The model under review builds one solid part; all positions refer to its coordinate system, in mm. A direction names the side the tool comes from. Coordinates: 2 decimals unless noted, no trailing zeros. Order: outer loops, then holes, each group sorted by start corner. A loop starts at its lowest first (then second) coordinate and runs counter-clockwise, first axis right, second up.
from build123d import *

# Parameters (mm, degrees)
EXTRUDE_1_DEPTH             = 15
HOLE_WIZARD_M121_D          = 10.2
HOLE_WIZARD_M121_DEPTH      = 15
HOLE_WIZARD_M61_D           = 5
HOLE_WIZARD_M61_DEPTH       = 15
HOLE_WIZARD_5_5_5_5_1_D     = 5.5
HOLE_WIZARD_5_5_5_5_1_DEPTH = 15
SKETCH_9_W                  = 6
SKETCH_9_H                  = 6
SKETCH_9_H_2                = 3
SKETCH_9_W_2                = 3
EXTRUDE_2_DEPTH             = 2
FILLET_1_R                  = 2


with BuildPart() as part:
    # Эскиз1 → Бобышка-Вытянуть1 (new body)
    with BuildSketch(Plane(origin=(0, 0, 0), x_dir=(1, 0, 0), z_dir=(0, 1, 0))):
        Polygon((0, 0), (0, 90), (30, 90), (90, 30), (90, 0), align=None)
    extrude(amount=EXTRUDE_1_DEPTH)

    # Отверстие обработанное метчиком M121
    with Locations(Plane(origin=(0, 15, 0), x_dir=(1, 0, 0), z_dir=(0, 1, 0))):
        with Locations((45, 45)):
            Hole(HOLE_WIZARD_M121_D / 2, depth=HOLE_WIZARD_M121_DEPTH)

    # Отверстие обработанное метчиком M61
    with Locations(Plane(origin=(0, 15, 0), x_dir=(1, 0, 0), z_dir=(0, 1, 0))):
        with Locations((37.928932188, 73.284271247), (73.284271247, 37.928932188), (52.071067812, 16.715728753), (16.715728753, 52.071067812)):
            Hole(HOLE_WIZARD_M61_D / 2, depth=HOLE_WIZARD_M61_DEPTH)

    # Диаметр отверстия Ø5.5 (5.5)1
    with Locations(Plane(origin=(0, 15, 0), x_dir=(1, 0, 0), z_dir=(0, 1, 0))):
        with Locations((15, 75), (15, 40), (15, 15), (40, 15), (75, 15)):
            Hole(HOLE_WIZARD_5_5_5_5_1_D / 2, depth=HOLE_WIZARD_5_5_5_5_1_DEPTH)

    # Эскиз9 → Бобышка-Вытянуть2 (add)
    with BuildSketch(Plane(origin=(0, 15, 0), x_dir=(1, 0, 0), z_dir=(0, 1, 0))):
        with Locations((15, 83)):
            Rectangle(SKETCH_9_W, SKETCH_9_H)
        with Locations((15, 60.071067812)):
            Rectangle(SKETCH_9_W, SKETCH_9_H)
        with Locations((15, 32)):
            Rectangle(SKETCH_9_W, SKETCH_9_H_2)
        with Locations((32, 15)):
            Rectangle(SKETCH_9_W_2, SKETCH_9_H)
        with Locations((60.071067812, 15)):
            Rectangle(SKETCH_9_W, SKETCH_9_H)
        with Locations((83, 15)):
            Rectangle(SKETCH_9_W, SKETCH_9_H)
    extrude(amount=EXTRUDE_2_DEPTH)

    # Скругление1
    fillet_1_edges = [part.edges().sort_by_distance(p)[0] for p in [
        (0, 7.5, 0),
        (0, 7.5, -90),
        (30, 7.5, -90),
        (90, 7.5, -30),
        (90, 7.5, 0),
    ]]
    fillet(fillet_1_edges, radius=FILLET_1_R)


solid = part.part
(1) Wall thickness on line 1 (X direction, y = 7.25, z = -15); line 2 (Z direction, x = 15, y = 3); line 3 (Y direction, x = 37.5, z = -39.5): over which ranges is each line inside the solid? List them lowest first.
(2) Insertion check: pin 1 Ø2 at (y, z) = (16.5, -14.5) entering from +X; pin 2 Ø8 at (x, z) = (16.72, -52.07) entering from +Y; pin 3 Ø0.6 at (x, y) = (15.5, 16) entering from +Z. Each pin has a flat end and moves straight along its axis. Give the tip position at first contact, or say it passes through.
(3) Consider section B-B (x = 41.5). Give the boundary of the cut face in (y, z).
(4) Consider section D-D (x = 59). Give the boundary of the cut face in (y, z).
(5) The part is to be moulded in two halves that separate along Z. For faces 1 (the face through (60, 7, -60)), 2 (the face through (15.358, 7.395, -17.727)), 3 (the face through (15.358, 7.395, -42.727)), 4 (the face through (36, 0, -36)), say which applies: +Z half, -Z half, draft (parallel to the pull), parting line (faces both ways), or undercut.
(6) Consider section A-A (z = -45). Give the boundary of the cut face in (x, y), then the cut area to 3 significant figures.
(7) Consider section C-C (y = 6.25). Give the number of separate pieces and of enclosed holes in the cut face, then the cut area to 3 significant figures.
(8) Tool access review of faces 5 (the face through (15, 16, -57.071)), 6 (the face through (18, 16, -83)), 7 (the face through (60, 16, -12)), 8 (the face through (15, 7, -90)), 9 (the face through (83, 16, -18)): name each direction out of +Z, -Z, +X, -X, +Y, -Y from which nothing blocks a thin tool from reaching the whole face with its end or side.
Findings:
1. line 1: x = 0 to 12.25, 17.75 to 37.25, 42.75 to 50.25, 53.89 to 72.25, 77.75 to 90
1. line 2: z = -90 to -77.75, -72.25 to -53.89, -50.25 to -42.75, -37.25 to -17.75, -12.25 to 0
1. line 3: y = 0 to 15
2. pin 1: stops at x = 86
2. pin 2: stops at y = 15
2. pin 3: stops at z = -30.5
3. outline: (0, -78.5) - (15, -78.5) - (15, -48.71) - (0, -48.71) - close; (0, -41.29) - (15, -41.29) - (15, -17.3) - (0, -17.3) - close; (0, -12.7) - (15, -12.7) - (15, 0) - (0, 0) - close
4. outline: (0, -61) - (15, -61) - (15, -18) - (17, -18) - (17, -12) - (15, -12) - (15, 0) - (0, 0) - close
5. face 1: -Z half
5. face 2: undercut
5. face 3: undercut
5. face 4: draft
6. outline: (0, 0) - (39.9, 0) - (39.9, 15) - (0, 15) - close; (50.1, 0) - (75, 0) - (75, 15) - (50.1, 15) - close
6. area: 972 mm2
7. separate pieces: 1
7. enclosed holes: 10
7. area: 6,020 mm2
8. face 5: +X, -X, +Y
8. face 6: +Z, -Z, +X, +Y
8. face 7: +Z, +X, -X, +Y
8. face 8: -Z, +X, -X, +Y, -Y
8. face 9: -Z, +X, -X, +Y
